Verification items for the finished model (mm, model axes). A direction names the side the tool comes from. Give positions to 0.01 mm unless a question says otherwise; leave off trailing zeros. Write each loop counter-clockwise with the first axis right and the second up, starting at its lowest first coordinate (ties: lowest second). Pieces come first, ordered by that corner, then holes.
from build123d import *

# Parameters (mm, degrees)
SKETCH_1_W          = 23.5
SKETCH_1_H          = 53
SKETCH_1_W_2        = 20.1
SKETCH_1_H_2        = 49.6
EXTRUDE_1_DEPTH     = 7
SKETCH_1_5_R        = 1.25
EXTRUDE_2_DEPTH     = 7
SKETCH_1_6_R        = 1.25
SKETCH_1_6_W        = 20.1
SKETCH_1_6_H        = 49.6
EXTRUDE_3_DEPTH     = 2
SKETCH_2_W          = 13.2
SKETCH_2_H          = 1.7
SKETCH_2_W_2        = 12
CUT_EXTRUDE_1_DEPTH = 3
SKETCH_2_3_R        = 0.65
EXTRUDE_4_DEPTH     = 2
FILLET_1_R          = 1.5


with BuildPart() as part:
    # Sketch 1 → Extrude 1 (new body)
    with BuildSketch(Plane.XY):
        with Locations((11.75, -26.5)):
            Rectangle(SKETCH_1_W, SKETCH_1_H)
        with Locations((11.75, -26.5)):
            Rectangle(SKETCH_1_W_2, SKETCH_1_H_2, mode=Mode.SUBTRACT)
    extrude(amount=EXTRUDE_1_DEPTH)

    # Sketch 1_5 → Extrude 2 (add)
    with BuildSketch(Plane.XY):
        with Locations((1.25, -26.7)):
            Circle(SKETCH_1_5_R)
        with Locations((22.25, -26.7)):
            Circle(SKETCH_1_5_R)
    extrude(amount=EXTRUDE_2_DEPTH)

    # Sketch 1_6 → Extrude 3 (add)
    with BuildSketch(Plane.XY):
        with Locations((22.25, -26.7)):
            Circle(SKETCH_1_6_R)
        with Locations((1.25, -26.7)):
            Circle(SKETCH_1_6_R)
        with Locations((11.75, -26.5)):
            Rectangle(SKETCH_1_6_W, SKETCH_1_6_H)
    extrude(amount=EXTRUDE_3_DEPTH)

    # Sketch 2 → Cut-Extrude 1 (cut)
    with BuildSketch(Plane.XY.offset(7)):
        with Locations((11.75, -52.15)):
            Rectangle(SKETCH_2_W, SKETCH_2_H)
        with Locations((11.75, -0.85)):
            Rectangle(SKETCH_2_W_2, SKETCH_2_H)
    extrude(amount=-CUT_EXTRUDE_1_DEPTH, mode=Mode.SUBTRACT)

    # Sketch 2_3 → Extrude 4 (add)
    with BuildSketch(Plane.XY.offset(7)):
        with Locations((22.25, -26.7)):
            Circle(SKETCH_2_3_R)
        with Locations((1.25, -26.7)):
            Circle(SKETCH_2_3_R)
    extrude(amount=EXTRUDE_4_DEPTH)

    # Fillet 1
    fillet_1_edges = [part.edges().sort_by_distance(p)[0] for p in [
        (0, -13.35, 0),
        (11.75, 0, 0),
        (23.5, -13.35, 0),
        (11.75, -53, 0),
        (0, -53, 3.5),
        (0, 0, 3.5),
        (23.5, 0, 3.5),
        (23.5, -53, 3.5),
    ]]
    fillet(fillet_1_edges, radius=FILLET_1_R)


solid = part.part
Item 1: Sectioned sample at A-A on z = 4.75. Record the cut outline in (x, y), then the cut area to 3 significant figures.
Answer key:
outline: (0, -51.5) arc R1.5 ccw to (1.5, -53) - (5.15, -53) - (5.15, -51.3) - (1.7, -51.3) - (1.7, -27.87) arc R1.25 ccw to (1.7, -25.53) - (1.7, -1.7) - (5.75, -1.7) - (5.75, 0) - (1.5, 0) arc R1.5 ccw to (0, -1.5) - close; (17.75, -1.7) - (21.8, -1.7) - (21.8, -25.53) arc R1.25 ccw to (21.8, -27.87) - (21.8, -51.3) - (18.35, -51.3) - (18.35, -53) - (22, -53) arc R1.5 ccw to (23.5, -51.5) - (23.5, -1.5) arc R1.5 ccw to (22, 0) - (17.75, 0) - close
area: 206 mm2
Item 2: Scan lines: line 1 along Y through (x, z) = (10.5, 2.75); line 2 along X through (y, z) = (-12, 3); line 3 along Z through (x, y) = (11.25, -8). Record each from-to range of solid material in increasing order.
Answer key:
line 1: y = -53 to -51.3, -1.7 to 0
line 2: x = 0 to 1.7, 21.8 to 23.5
line 3: z = 0 to 2
Item 3: Sectioned sample at B-B on y = -26.7. Record the cut outline in (x, z), then the cut area to 3 significant figures.
Answer key:
outline: (0, 1.5) arc R1.5 ccw to (1.5, 0) - (22, 0) arc R1.5 ccw to (23.5, 1.5) - (23.5, 7) - (22.9, 7) - (22.9, 9) - (21.6, 9) - (21.6, 7) - (21, 7) - (21, 2) - (2.5, 2) - (2.5, 7) - (1.9, 7) - (1.9, 9) - (0.6, 9) - (0.6, 7) - (0, 7) - close
area: 76.2 mm2
Item 4: Set-up check for faces 1 (the face through (1, -27, 9)), 2 (the face through (17.75, -1, 6)), 3 (the face through (12, -51.3, 3)): record each of +Z, -Z, +X, -X, +Y, -Y from which the full face is reachable in a straight line by a thin tool's end or side.
Answer key:
face 1: +Z, +X, -X, +Y, -Y
face 2: +Z, +Y, -Y
face 3: +Z
Item 5: Depth check by flat-ended pin: pin 1 (1.4 mm diameter, centred on x = 13, y = -52, fed in from +Z); pin 2 (4.5 mm diameter, centred on x = 3, y = -19, fed in from +Z); pin 3 (4.5 mm diameter, centred on x = 19.5, y = -38, fed in from +Z). Enter the tip coordinate at first touch or a pass-through.
Answer key:
pin 1: stops at z = 4
pin 2: stops at z = 7
pin 3: stops at z = 2
Item 6: Release check for a two-part mould opening along X. For faces 4 (the face through (0.45, -26.15, 0.43)), 5 (the face through (23.05, -26.85, 0.43)), 6 (the face through (22, -27, 9)), 7 (the face through (5.15, -52, 6)) record: released by +X, released by -X, zero draft, split by the parting line, or undercut.
Answer key:
face 4: released by -X
face 5: released by +X
face 6: zero draft
face 7: undercut
Item 7: Sectioned sample at D-D on y = -15. Record the cut outline in (x, z).
Answer key:
outline: (0, 1.5) arc R1.5 ccw to (1.5, 0) - (22, 0) arc R1.5 ccw to (23.5, 1.5) - (23.5, 7) - (21.8, 7) - (21.8, 2) - (1.7, 2) - (1.7, 7) - (0, 7) - close
Item 8: Sectioned sample at C-C on x = 13.25. Record the cut outline in (y, z).
Answer key:
outline: (-53, 1.5) arc R1.5 ccw to (-51.5, 0) - (-1.5, 0) arc R1.5 ccw to (0, 1.5) - (0, 4) - (-1.7, 4) - (-1.7, 2) - (-51.3, 2) - (-51.3, 4) - (-53, 4) - close
